Check sheet for the modelled part. Datum: model origin and axes. Units: mm. Give positions to 0.01 mm unless a question says otherwise; leave off trailing zeros. Loops run counter-clockwise (first coordinate to the right, second up) from the corner with the lowest first, then second, coordinate; pieces in that order, holes last. Notation, with made-up numbers: (-32.5, 77.5) - (15.5, 77.5) arc R36 ccw to (15.5, 115.5) - close; hole circle Ø7 at (12, 30.5). An arc over 180 degrees is marked (long way). Use CSV: the item, a comma, the result in double quotes.
Autodesk Inventor part; units mm, degrees
ref_plane "YZ Plane" through (0, 0, 0) normal (1, 0, 0) x (0, 1, 0)
ref_plane "XZ Plane" through (0, 0, 0) normal (0, 1, 0) x (-1, 0, 0)
ref_plane "XY Plane" through (0, 0, 0) normal (0, 0, 1) x (1, 0, 0)
sketch "Skizze1" plane through (0, 0, 0) normal (0, 0, 1) x (1, 0, 0)
  circle A0 centre (0, 0) radius 38
  circle A1 centre (0, 0) radius 48
  dimension "d0" = 76
  dimension "d1" = 10
extrude "Extrusion1" add sketch "Skizze1" along normal blind 6
sketch "Skizze3" plane through (0, 0, 6) normal (0, 0, 1) x (1, 0, 0)
  circle A0 centre (0, 0) radius 40
  circle A1 centre (0, 0) radius 46
  circle A2 centre (0, 0) radius 38
  circle A3 centre (0, 0) radius 48
  dimension "d8" = 2
  dimension "d9" = 2
extrude "Extrusion3" cut sketch "Skizze3" against normal blind 2 contours A1
sketch "Skizze5" plane through (0, 0, 4) normal (0, 0, 1) x (1, 0, 0)
  circle A0 centre (0, 0) radius 46
  line L0 (0, 46) -> (0, 40)
  circle A1 centre (0, 0) radius 40
  circle A2 centre (0, 43) radius 2.5
  dimension "d12" = 5
extrude "Extrusion4" cut sketch "Skizze5" against normal blind 3 contours A2 L0 | L0 A2
pattern_circular "Runde Anordnung1" count 12 over 360 about axis through (0, 0, -10) along (0, 0, 1) of "Extrusion4"
properties part number "P_magnetCase" material "ABS-Kunststoff"
1. Sectioned sample at C-C, the plane y = 16. Record the boundary of the cut face in (x, z).
Completed:
outline,"(-45.25, 0) - (-34.47, 0) - (-34.47, 6) - (-36.66, 6) - (-36.66, 4) - (-43.13, 4) - (-43.13, 6) - (-45.25, 6) - close; (34.47, 0) - (45.25, 0) - (45.25, 6) - (43.13, 6) - (43.13, 4) - (36.66, 4) - (36.66, 6) - (34.47, 6) - close"
2. Sectioned sample at B-B, the plane x = -21.5. Record the boundary of the cut face in (y, z), and give its area (3 significant figures).
Completed:
outline,"(-42.92, 0) - (-31.33, 0) - (-31.33, 6) - (-33.73, 6) - (-33.73, 4) - (-34.74, 4) - (-34.74, 1) - (-39.74, 1) - (-39.74, 4) - (-40.67, 4) - (-40.67, 6) - (-42.92, 6) - close; (31.33, 0) - (42.92, 0) - (42.92, 6) - (40.67, 6) - (40.67, 4) - (39.74, 4) - (39.74, 1) - (34.74, 1) - (34.74, 4) - (33.73, 4) - (33.73, 6) - (31.33, 6) - close"
area,"81.2 mm²"
3. Sectioned sample at D-D, the plane y = 43. Record the boundary of the cut face in (x, z).
Completed:
outline,"(-21.33, 0) - (21.33, 0) - (21.33, 6) - (16.34, 6) - (16.34, 4) - (2.5, 4) - (2.5, 1) - (-2.5, 1) - (-2.5, 4) - (-16.34, 4) - (-16.34, 6) - (-21.33, 6) - close"
4. Scan lines: line 1 along Y through (x, z) = (-7, 5.55); line 2 along Y through (x, z) = (-26, 4.4); line 3 along X through (y, z) = (27, 4.9). Record each from-to range of solid material in increasing order.
Completed:
line 1,"y = -47.49 to -45.46, -39.38 to -37.35, 37.35 to 39.38, 45.46 to 47.49"
line 2,"y = -40.35 to -37.95, -30.4 to -27.71, 27.71 to 30.4, 37.95 to 40.35"
line 3,"x = -39.69 to -37.24, -29.51 to -26.74, 26.74 to 29.51, 37.24 to 39.69"
5. Release check for a two-part mould opening along Y. For faces 1 (the face through (37, 22, 1)), 2 (the face through (25, -39, 6)) record: released by +Y, released by -Y, zero draft, split by the parting line, or undercut.
Completed:
face 1,"undercut"
face 2,"zero draft"
6. Go/stop test with flat-tipped pins: pin 1 Ø4 at (x, y) = (-37.24, 21.5) entering from +Z; pin 2 Ø2.5 at (x, y) = (-36, 22.5) entering from +Z; pin 3 Ø2 at (x, z) = (-23.5, 5.5) entering from -Y. Record where each tip stops, or that it passes through.
Completed:
pin 1,"stops at z = 1"
pin 2,"stops at z = 4"
pin 3,"stops at y = -42.4"
7. Sectioned sample at A-A, the plane y = 5.5. Record the boundary of the cut face in (x, z), and give its area (3 significant figures).
Completed:
outline,"(-47.68, 0) - (-37.6, 0) - (-37.6, 6) - (-39.62, 6) - (-39.62, 4) - (-45.67, 4) - (-45.67, 6) - (-47.68, 6) - close; (37.6, 0) - (47.68, 0) - (47.68, 6) - (45.67, 6) - (45.67, 4) - (39.62, 4) - (39.62, 6) - (37.6, 6) - close"
area,"96.8 mm²"
